from build123d import *

# Parameters (mm, degrees)
SKETCH1_R           = 12.7
SKETCH1_R_2         = 4.7625
BOSS_EXTRUDE1_DEPTH = 3.175


with BuildPart() as part:
    # Sketch1 → Boss-Extrude1 (new body)
    with BuildSketch(Plane.XY):
        with BuildLine():
            Line((-12.70002942, 34.924992178), (-17.381139802, 34.924992178))
            Line((-17.381139802, 34.924992178), (-17.381139802, 15.948235146))
            Line((-17.381139802, 15.948235146), (-12.273648862, -3.263057403))
            ThreePointArc((-12.273648862, -3.263057403), (-1.645396526, 12.59296114), (12.7, 0))
            ThreePointArc((12.7, 0), (12.592963493, -1.645378514), (12.273658196, -3.263022292))
            Line((12.273658196, -3.263022292), (17.381080961, 15.948235146))
            Line((17.381080961, 15.948235146), (17.381080961, 34.924992178))
            Line((17.381080961, 34.924992178), (12.69997058, 34.924992178))
            ThreePointArc((12.69997058, 34.924992178), (-2.942e-05, 22.224992178), (-12.70002942, 34.924992178))
        make_face()
        Circle(SKETCH1_R)
        Circle(SKETCH1_R_2, mode=Mode.SUBTRACT)
    extrude(amount=BOSS_EXTRUDE1_DEPTH)


solid = part.part
The listing builds one solid part. Answer for the finished solid, in the listing's coordinates (mm). Give positions to 0.01 mm unless a question says otherwise; leave off trailing zeros. Write each loop counter-clockwise with the first axis right and the second up, starting at its lowest first coordinate (ties: lowest second). Pieces come first, ordered by that corner, then holes. Notation, with made-up numbers: (-10, -3.75) - (13, -3.75) arc R28 ccw to (13, 15.25) - close; hole circle Ø3 at (10.25, 39.5). An arc over 180 degrees is marked (long way). One line per question, with ' | ' between items. Start each with the question number.
1. Section B-B, the plane z = 0.5 is taken. Determine the outline of the cut face in (x, y) (1 decimal).
2. Section D-D, the plane y = -6 is taken. Determine the outline of the cut face in (x, z) (3 decimals), then the cut area to 3 significant figures.
3. Section A-A, the plane x = 0 is taken. Determine the outline of the cut face in (y, z) (1 decimal), then the cut area to 3 significant figures.
4. Determine the mould class of faces 1 (the face through (-0.2, -12.7, 1.6)), 2 (the face through (0, 11, 0)), 3 (the face through (-3.78, -2.9, 1.57)), 4 (the face through (-15, 34.925, 2)) for opening direction Y: +Y half, -Y half, draft (parallel to the pull), parting line (faces both ways), or undercut.
5. Section C-C, the plane y = 0 is taken. Determine the outline of the cut face in (x, z) (1 decimal).
6. Straight lines are drawn through the part: line 1 (Y direction, x = 0, z = 1.4) (1 decimal); line 2 (X direction, y = 31, z = 2.7); line 3 (Y direction, x = 0.5, z = 0.85). For each, find the intervals that lie inside material, in ascending order.
Result:
1) outline: (-17.4, 15.9) - (-12.3, -3.3) arc R12.7 ccw to (12.3, -3.3) - (17.4, 15.9) - (17.4, 34.9) - (12.7, 34.9) arc R12.7 cw to (-12.7, 34.9) - (-17.4, 34.9) - close; hole circle Ø9.5 at (0, 0)
2) outline: (-11.193, 0) - (11.193, 0) - (11.193, 3.175) - (-11.193, 3.175) - close | area: 71.1 mm2
3) outline: (-12.7, 0) - (-4.8, 0) - (-4.8, 3.2) - (-12.7, 3.2) - close; (4.8, 0) - (22.2, 0) - (22.2, 3.2) - (4.8, 3.2) - close | area: 80.6 mm2
4) face 1: -Y half | face 2: draft | face 3: undercut | face 4: +Y half
5) outline: (-13.1, 0) - (-4.8, 0) - (-4.8, 3.2) - (-13.1, 3.2) - close; (4.8, 0) - (13.1, 0) - (13.1, 3.2) - (4.8, 3.2) - close
6) line 1: y = -12.7 to -4.8, 4.8 to 22.2 | line 2: x = -17.38 to -12.08, 12.08 to 17.38 | line 3: y = -12.69 to -4.74, 4.74 to 22.23
